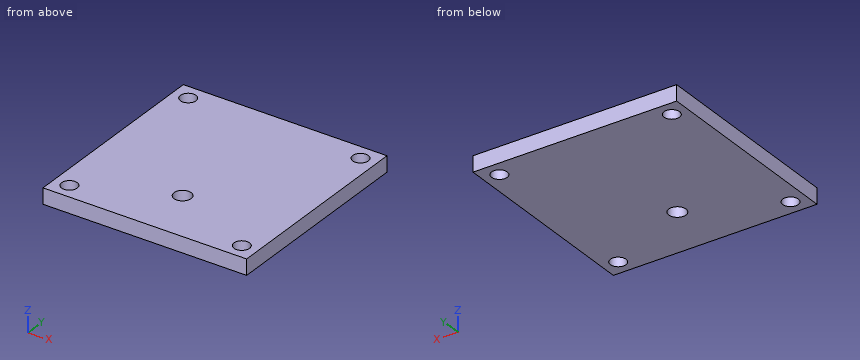
Autodesk Inventor part; units mm, degrees
ref_plane "YZ Plane" through (0, 0, 0) normal (1, 0, 0) x (0, 1, 0)
ref_plane "XZ Plane" through (0, 0, 0) normal (0, 1, 0) x (-1, 0, 0)
ref_plane "XY Plane" through (0, 0, 0) normal (0, 0, 1) x (1, 0, 0)
sketch "Sketch1" plane through (0, 0, 0) normal (0, 0, 1) x (1, 0, 0)
  line L0 (0, 0) -> (130, 0)
  line L1 (130, 0) -> (130, 130)
  line L2 (130, 130) -> (0, 130)
  line L3 (0, 130) -> (0, 0)
  dimension "d0" = 130
  dimension "d1" = 130
extrude "Extrusion1" add sketch "Sketch1" along normal blind 10
sketch "Sketch2" plane through (0, 0, 10) normal (0, 0, 1) x (1, 0, 0)
  line L0 (130, 130) -> (0, 130)
  line L1 (0, 130) -> (10, 130)
  line L2 (10, 130) -> (10, 0)
  line L3 (10, 0) -> (120, 0)
  line L4 (0, 0) -> (130, 0)
  line L5 (120, 0) -> (120, 130)
  line L6 (120, 130) -> (120, 120)
  line L7 (120, 120) -> (10, 120)
  line L8 (130, 0) -> (130, 10)
  line L9 (130, 0) -> (130, 130)
  line L10 (130, 10) -> (0, 10)
  line L11 (0, 130) -> (0, 0)
  circle A0 centre (10, 120) radius 5
  circle A1 centre (120, 120) radius 5
  circle A2 centre (120, 10) radius 5
  circle A3 centre (10, 10) radius 5
  dimension "d4" = 10
  dimension "d5" = 130
  dimension "d6" = 110
  dimension "d7" = 10
  dimension "d8" = 10
  dimension "d9" = 130
  dimension "d10" = 10
  dimension "d11" = 10
  dimension "d12" = 10
  dimension "d13" = 10
extrude "Extrusion2" cut sketch "Sketch2" against normal through all contours A1 L5 | L5 L7 A1 | A2 L5 L10 | L10 L5 A2 | A0 L7 L2 | L2 A0 | L5 A1 L7 | L10 A2 L5 | L5 A2 L10 | L7 A0 L2 | A3 L2 L10 | L10 L2 A3 | A3 L10 L2 | L2 L10 A3
sketch "Sketch3" plane through (0, 0, 10) normal (0, 0, 1) x (1, 0, 0)
  line L0 (0, 0) -> (130, 0)
  line L1 (65, 0) -> (30, 0)
  line L2 (65, 0) -> (65, 35)
  circle A0 centre (65, 35) radius 5.5
  dimension "d16" = 65
  dimension "d17" = 35
  dimension "d18" = 35
  dimension "d19" = 11
extrude "Extrusion3" cut sketch "Sketch3" against normal through all
thread "Thread1"
properties part number "2"
Design review of the part built by this model. Coordinates are the model's own, in mm. Coordinates: 2 decimals unless noted, no trailing zeros. Loops run counter-clockwise (first coordinate to the right, second up) from the corner with the lowest first, then second, coordinate; pieces in that order, holes last.
Item 1: Add section B-B (y = 120). Write out the cut boundary in (x, z).
Completed:
outline: (0, 0) - (5, 0) - (5, 10) - (0, 10) - close; (15, 0) - (115, 0) - (115, 10) - (15, 10) - close; (125, 0) - (130, 0) - (130, 10) - (125, 10) - close
Item 2: Add section C-C (z = 6.75). Write out the cut boundary in (x, y).
Completed:
outline: (0, 0) - (130, 0) - (130, 130) - (0, 130) - close; hole circle Ø10 at (10, 10); hole circle Ø10 at (10, 120); hole circle Ø11 at (65, 35); hole circle Ø10 at (120, 10); hole circle Ø10 at (120, 120)
Item 3: Wall thickness on L1, parallel to X at y = 120, z = 7.5; L2, parallel to Y at x = 118, z = 4.75: over which ranges is each line inside the solid? List them lowest first.
Completed:
L1: x = 0 to 5, 15 to 115, 125 to 130
L2: y = 0 to 5.42, 14.58 to 115.42, 124.58 to 130
Item 4: Clearance check with flat-ended pins moving along their axes: pin 1 (3 mm diameter, centred on y = 85.5, z = 5.5, fed in from -X); pin 2 (9 mm diameter, centred on x = 10, y = 120, fed in from -Z). State where each tip first meets the part, or that it passes through.
Completed:
pin 1: stops at x = 0
pin 2: passes through
Item 5: Add section A-A (y = 35). Write out the cut boundary in (x, z).
Completed:
outline: (0, 0) - (59.5, 0) - (59.5, 10) - (0, 10) - close; (70.5, 0) - (130, 0) - (130, 10) - (70.5, 10) - close
